Work out the finished part from the listing and answer in its coordinate system (mm). Face numbers are marked on the shaded views. Give positions to 0.01 mm unless a question says otherwise; leave off trailing zeros. Write each loop counter-clockwise with the first axis right and the second up, starting at its lowest first coordinate (ties: lowest second). Pieces come first, ordered by that corner, then holes. Notation, with made-up numbers: (29, 72) -> (50, 72) arc R19 ccw to (50, 104) -> close; hole circle Ø5 at (36, 37.5). An arc over 180 degrees is marked (long way). Use a Markdown table: item, result. Add a question column.
Q1. For a pull along Y with two mould halves and no side action, classify the marked faces 1 and 2 as pulls with the +Y half, pulls with the -Y half, needs draft (parallel to the pull), parting line crosses it, or undercut.
Q2. Each of these flat-tipped pins is pushed along its axis until it touches: pin 1 Ø1.5 at (y, z) = (4.5, 43.5) entering from +X; pin 2 Ø1.5 at (y, z) = (2.5, 32.5) entering from +X; pin 3 Ø5 at (x, z) = (-32, -1) entering from +Y. Where does it stop, or does it pass through?
Q3. Section B-B, the plane x = 25.5 is taken. Give the vertices of the cut face in (y, z), plus the area to 3 significant figures.
Q4. Section C-C, the plane y = 3.25 is taken. Give the vertices of the cut face in (x, z), plus the area to 3 significant figures.
Q5. Consider line 1 (X direction, y = 4.35, z = 0); line 2 (Z direction, x = 26, y = 5); line 3 (Z direction, x = 17.5, y = 6). Determine where each line is inside the solid, lowest interval first.
Q6. Section D-D, the plane z = 41 is taken. Give the vertices of the cut face in (x, y).
Q7. Section A-A, the plane z = 0 is taken. Give the vertices of the cut face in (x, y), plus the area to 3 significant figures.
from build123d import *

# Parameters (mm, degrees)
SKETCH1_R             = 100
BOSS_EXTRUDE1_DEPTH   = 7
SKETCH2_R             = 5
CUT_EXTRUDE1_DEPTH    = 142.594491418
SKETCH3_R             = 8.479886046
CUT_EXTRUDE2_DEPTH    = 5.482684
CIRPATTERN1_START     = 1.517316099
CIRPATTERN1_OUTLINE_R = 8.479886046
CIRPATTERN1_DEPTH     = 5.482683901


# Read off the part's stored shape, not the designer's step: CirPattern1
with BuildPart() as part:
    # Sketch1 → Boss-Extrude1 (new body)
    with BuildSketch(Plane(origin=(0, 0, 0), x_dir=(1, 0, 0), z_dir=(0, 1, 0))):
        with Locations(Location((0, 0, 0), (0, 0, 270))):
            Circle(SKETCH1_R)
    extrude(amount=BOSS_EXTRUDE1_DEPTH)

    # Sketch2 → Cut-Extrude1 (cut, through all)
    with BuildSketch(Plane(origin=(0, 0, 0), x_dir=(1, 0, 0), z_dir=(0, 1, 0))):
        with Locations(Location((0, 0, 0), (0, 0, 270))):
            Circle(SKETCH2_R)
    extrude(amount=CUT_EXTRUDE1_DEPTH, mode=Mode.SUBTRACT)

    # Sketch3 → Cut-Extrude2 (cut)
    with BuildSketch(Plane(origin=(0, 7, 0), x_dir=(1, 0, 0), z_dir=(0, 1, 0))):
        with Locations(Location((-31.267640686, 0, 0), (0, 0, 270))):
            Circle(SKETCH3_R)
    extrude(amount=-CUT_EXTRUDE2_DEPTH, mode=Mode.SUBTRACT)

    # CirPattern1 outline → CirPattern1 (cut)
    with BuildSketch(Plane(origin=(0, 0, 0), x_dir=(1, 0, 0), z_dir=(0, 1, 0)).offset(CIRPATTERN1_START)):
        with Locations((-9.662232346, -29.737293423)):
            Circle(CIRPATTERN1_OUTLINE_R)
        with Locations((25.296052689, -18.378658069)):
            Circle(CIRPATTERN1_OUTLINE_R)
        with Locations((25.296052689, 18.378658069)):
            Circle(CIRPATTERN1_OUTLINE_R)
        with Locations((-9.662232346, 29.737293423)):
            Circle(CIRPATTERN1_OUTLINE_R)
    extrude(amount=CIRPATTERN1_DEPTH, mode=Mode.SUBTRACT)


solid = part.part
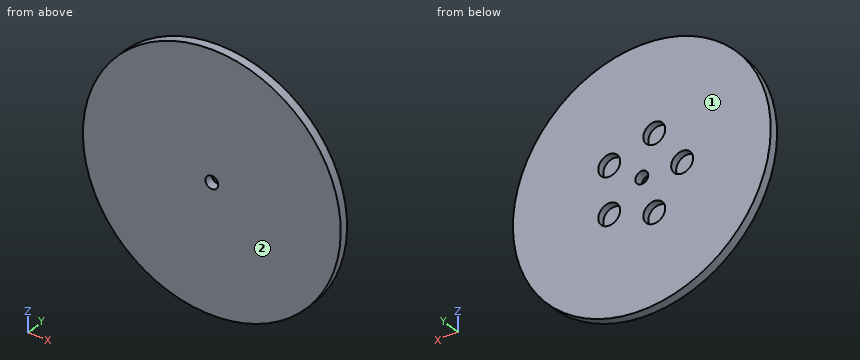
Result set:
| question | item | result |
|---|---|---|
| 1 | face 1 | pulls with the +Y half |
| 1 | face 2 | pulls with the -Y half |
| 2 | pin 1 | stops at x = 90.4 |
| 2 | pin 2 | stops at x = 94.83 |
| 2 | pin 3 | stops at y = 1.52 |
| 3 | outline | (0, -96.69) -> (7, -96.69) -> (7, -26.86) -> (1.52, -26.86) -> (1.52, -9.9) -> (7, -9.9) -> (7, 9.9) -> (1.52, 9.9) -> (1.52, 26.86) -> (7, 26.86) -> (7, 96.69) -> (0, 96.69) -> close |
| 3 | area | 1,170 mm2 |
| 4 | outline | circle Ø200 at (0, 0); hole circle Ø16.96 at (-31.27, 0); hole circle Ø16.96 at (-9.66, -29.74); hole circle Ø16.96 at (-9.66, 29.74); hole circle Ø10 at (0, 0); hole circle Ø16.96 at (25.3, -18.38); hole circle Ø16.96 at (25.3, 18.38) |
| 4 | area | 30,200 mm2 |
| 5 | line 1 | x = -100 to -39.75, -22.79 to -5, 5 to 100 |
| 5 | line 2 | z = -96.56 to -26.83, -9.93 to 9.93, 26.83 to 96.56 |
| 5 | line 3 | z = -98.46 to -21.71, -15.04 to 15.04, 21.71 to 98.46 |
| 6 | outline | (-91.21, 0) -> (91.21, 0) -> (91.21, 7) -> (-91.21, 7) -> close |
| 7 | outline | (-100, 0) -> (-5, 0) -> (-5, 7) -> (-22.79, 7) -> (-22.79, 1.52) -> (-39.75, 1.52) -> (-39.75, 7) -> (-100, 7) -> close; (5, 0) -> (100, 0) -> (100, 7) -> (5, 7) -> close |
| 7 | area | 1,240 mm2 |
